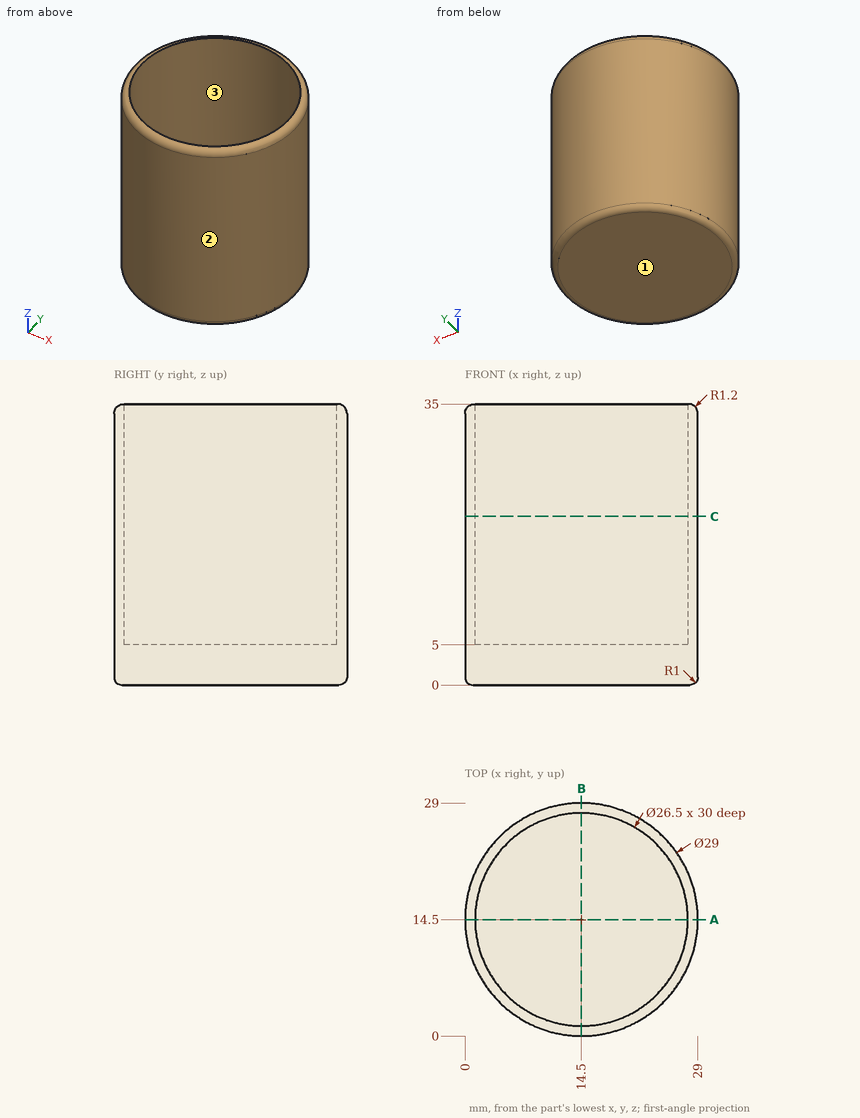
For this review, use the dimensioned drawing (mm, ordinates from the lowest corner) and the shaded views. Give positions to 0.01 mm unless a question says otherwise; leave off trailing zeros. Order: outer loops, then holes, each group sorted by start corner. A loop starts at its lowest first (then second) coordinate and runs counter-clockwise, first axis right, second up.
1) The part is to be moulded in two halves that separate along X. For the marked faces 1, 2 and 3, say which applies: released by +X, released by -X, zero draft, split by the parting line, or undercut.
2) Take a section at A-A (y = 14.5). Give the boundary of the cut face in (x, z).
3) Wall thickness on line 1 (Y direction, x = 14.5, z = 22.5); line 2 (Y direction, x = 5.5, z = 27); line 3 (X direction, y = 4.75, z = 32): over which ranges is each line inside the solid? List them lowest first.
4) Take a section at C-C (z = 21). Give the boundary of the cut face in (x, y).
5) Insertion check: pin 1 (1 mm diameter, centred on y = 11, z = 15, fed in from +X); pin 2 (1.5 mm diameter, centred on x = 19.5, z = 26, fed in from -Y); pin 3 (8 mm diameter, centred on x = 14, y = 9.5, fed in from +Z). Each pin has a flat end and moves straight along its axis. Give the tip position at first contact, or say it passes through.
Derived:
1. face 1: zero draft
1. face 2: split by the parting line
1. face 3: undercut
2. outline: (0, 1) arc R1 ccw to (1, 0) - (28, 0) arc R1 ccw to (29, 1) - (29, 33.8) arc R1.2 ccw to (27.8, 35) - (27.75, 35) - (27.75, 5) - (1.25, 5) - (1.25, 35) - (1.2, 35) arc R1.2 ccw to (0, 33.8) - close
3. line 1: y = 0 to 1.25, 27.75 to 29
3. line 2: y = 3.13 to 4.78, 24.22 to 25.87
3. line 3: x = 3.77 to 5.53, 23.47 to 25.23
4. outline: circle Ø29 at (14.5, 14.5); hole circle Ø26.5 at (14.5, 14.5)
5. pin 1: stops at x = 28.69
5. pin 2: stops at y = 0.64
5. pin 3: stops at z = 5
